The listing builds one solid part. Answer for the finished solid, in the listing's coordinates (mm). A direction names the side the tool comes from. Coordinates: 2 decimals unless noted, no trailing zeros. Order: outer loops, then holes, each group sorted by start corner. A loop starts at its lowest first (then second) coordinate and runs counter-clockwise, first axis right, second up. Notation, with made-up numbers: (0.25, -17) -> (57.25, -17) arc R13 ccw to (57.25, -11) -> close; hole circle Ø10 at (47, 39). An arc over 180 degrees is marked (long way). Return JSON: item names as keys, results as strings.
```python
from build123d import *

# Parameters (mm, degrees)
SKETCH1_W               = 38.1
SKETCH1_H               = 33.86758938
BOSS_EXTRUDE1_DEPTH     = 12.7
F_1_4_CLEARANCE_HOLE1_D = 7.14248
HOLE1_AT_2_COUNT        = 2
HOLE1_AT_2_PITCH        = 20.32
SKETCH9_W               = 9.525
SKETCH9_H               = 6.35
CUT_EXTRUDE1_DEPTH      = 34.86758938
CHAMFER1_SIZE           = 2.54
CHAMFER2_SIZE           = 1.27


with BuildPart() as part:
    # Sketch1 → Boss-Extrude1 (new body)
    with BuildSketch(Plane.XY):
        with Locations((-124.004465969, 21.4125)):
            Rectangle(SKETCH1_W, SKETCH1_H)
    extrude(amount=BOSS_EXTRUDE1_DEPTH)

    # 1/4 Clearance Hole1 (through all)
    with Locations(Plane(origin=(0, 0, 0), x_dir=(-1, 0, 0), z_dir=(0, 0, -1))):
        with Locations((124.004465969, 11.2525), (124.004465969, 31.5725)):
            Hole(F_1_4_CLEARANCE_HOLE1_D / 2)

    # Sketch8 → Hole1 (revolve, cut)
    with BuildSketch(Plane(origin=(-124.004465969, 11.2525, 12.7), x_dir=(0, -1, 0), z_dir=(1, 0, 0))):
        Polygon((0, 0), (0, 7.62), (4.4323, 7.62), (4.6101, 0), align=None)
    hole1 = revolve(axis=Axis((-124.004465969, 11.2525, -97.3), (0, 0, 1)), mode=Mode.SUBTRACT)

    # Hole1 at 2: Hole1 ×2
    with Locations(*[(0, i * HOLE1_AT_2_PITCH, 0) for i in range(1, HOLE1_AT_2_COUNT)]):
        add(hole1, mode=Mode.SUBTRACT)

    # Sketch9 → Cut-Extrude1 (cut, through all)
    with BuildSketch(Plane.XZ.offset(-4.47870531)):
        with Locations((-109.716965969, 9.525)):
            Rectangle(SKETCH9_W, SKETCH9_H)
        with Locations((-138.291965969, 9.525)):
            Rectangle(SKETCH9_W, SKETCH9_H)
    extrude(amount=-CUT_EXTRUDE1_DEPTH, mode=Mode.SUBTRACT)

    # Chamfer1
    chamfer1_edges = [part.edges().sort_by_distance(p)[0] for p in [
        (-143.054465969, 38.34629469, 3.175),
        (-104.954465969, 38.34629469, 3.175),
        (-104.954465969, 4.47870531, 3.175),
        (-143.054465969, 4.47870531, 3.175),
        (-114.479465969, 21.4125, 6.35),
        (-133.529465969, 21.4125, 6.35),
    ]]
    chamfer(chamfer1_edges, length=CHAMFER1_SIZE)

    # Chamfer2
    chamfer2_edges = [part.edges().sort_by_distance(p)[0] for p in [
        (-143.054465969, 21.4125, 0),
        (-124.004465969, 38.34629469, 0),
        (-104.954465969, 21.4125, 0),
        (-124.004465969, 4.47870531, 0),
        (-106.224465969, 5.74870531, 0),
        (-141.784465969, 5.74870531, 0),
        (-106.224465969, 37.07629469, 0),
        (-141.784465969, 37.07629469, 0),
    ]]
    chamfer(chamfer2_edges, length=CHAMFER2_SIZE)


solid = part.part
```
Item 1: Find the intervals of material crossed by probe 1 along Y at (x, z) = (-123.5, 3); probe 2 along Y at (x, z) = (-122, 10.25); probe 3 along Z at (x, y) = (-111.5, 26), in increasing order.
Answer list:
{"probe 1": "4.48 to 7.72, 14.79 to 28.04, 35.11 to 38.35", "probe 2": "4.48 to 7.16, 15.34 to 27.48, 35.66 to 38.35", "probe 3": "0 to 6.35"}
Item 2: Flat-ended cylindrical pins translate along their axes: pin 1 (1.5 mm diameter, centred on y = 16, z = 8.5, fed in from -X); pin 2 (7.5 mm diameter, centred on x = -138, y = 23, fed in from +Z); pin 3 (2 mm diameter, centred on x = -108.5, y = 23.5, fed in from +Z). Find the tip coordinate at first contact, or state that the pin passes through.
Answer list:
{"pin 1": "x = -134.67", "pin 2": "z = 8.17", "pin 3": "z = 6.35"}
Item 3: Determine the mould class of faces 4 (the flat face through (-142.411, 21.211, 0.626)), 5 (the cylindrical face through (-127.572, 11.41, 2.576)), 6 (the flat face through (-106.21, 37.06, 3.77)) for opening direction Y: pulls with the +Y half, pulls with the -Y half, needs draft (parallel to the pull), parting line crosses it, or undercut.
Answer list:
{"face 4": "needs draft", "face 5": "undercut", "face 6": "pulls with the +Y half"}
Item 4: The part is cut by section C-C on x = -134. Determine the outline of the cut face in (y, z), plus the area to 3 significant figures.
Answer list:
{"outline": "(4.48, 1.27) -> (5.75, 0) -> (37.08, 0) -> (38.35, 1.27) -> (38.35, 8.42) -> (4.48, 8.42) -> close", "area": "284 mm2"}
Item 5: The part is cut by section B-B on z = 4.25. Determine the outline of the cut face in (x, y), plus the area to 3 significant figures.
Answer list:
{"outline": "(-143.05, 7.02) -> (-140.51, 4.48) -> (-107.49, 4.48) -> (-104.95, 7.02) -> (-104.95, 35.81) -> (-107.49, 38.35) -> (-140.51, 38.35) -> (-143.05, 35.81) -> close; hole circle Ø7.14 at (-124, 11.25); hole circle Ø7.14 at (-124, 31.57)", "area": "1,200 mm2"}
Item 6: The part is cut by section A-A on y = 18.5. Determine the outline of the cut face in (x, z).
Answer list:
{"outline": "(-143.05, 1.27) -> (-141.78, 0) -> (-106.22, 0) -> (-104.95, 1.27) -> (-104.95, 6.35) -> (-111.94, 6.35) -> (-114.48, 8.89) -> (-114.48, 12.7) -> (-133.53, 12.7) -> (-133.53, 8.89) -> (-136.07, 6.35) -> (-143.05, 6.35) -> close"}
Item 7: Which of the six approach directions +Z, -Z, +X, -X, +Y, -Y give full straight-line access (tool end or side, diameter ignored) to faces 1 (the flat face through (-140, 21, 6.35)), 2 (the flat face through (-124, 22, 12.7)), 3 (the flat face through (-120, 32, 5.08))?
Answer list:
{"face 1": "+Z, -X, +Y, -Y", "face 2": "+Z, +X, -X, +Y, -Y", "face 3": "+Z"}
Item 8: The part is cut by section D-D on x = -125.5. Count the separate pieces of the cut face and the enclosed holes in it, plus the area to 3 significant figures.
Answer list:
{"separate pieces": "3", "enclosed holes": "0", "area": "233 mm2"}
